from build123d import *
from build123d.topology import SkipClean

# Parameters (mm, degrees)
ESQUISSE1_W             = 22
ESQUISSE1_H             = 25
EXTRUSION1_DEPTH        = 5
EXTRUSION2_DEPTH        = 22
EXTRUSION3_DEPTH        = 9
EXTRUSION4_DEPTH        = 7.7
ESQUISSE6_R             = 1.25
EXTRUSION5_DEPTH        = 36
ENL_V_MAT_EXTRU_2_DEPTH = 6.678544503


with BuildPart() as part:
    # Esquisse1 → Extrusion1 (new, symmetric)
    with BuildSketch(Plane.XY):
        with Locations((11, 12.5)):
            Rectangle(ESQUISSE1_W, ESQUISSE1_H)
    extrude(amount=EXTRUSION1_DEPTH, both=True)

    # Esquisse2 → Extrusion2 (add)
    with BuildSketch(Plane.ZY):
        with BuildLine():
            Line((-5, 0), (5, 0))
            ThreePointArc((5, 0), (5.353553391, -0.146446609), (5.5, -0.5))
            Line((5.5, -0.5), (5.5, -10))
            Line((5.5, -10), (-5.5, -10))
            Line((-5.5, -10), (-5.5, -0.5))
            ThreePointArc((-5.5, -0.5), (-5.353553391, -0.146446609), (-5, 0))
        make_face()
    extrude(amount=-EXTRUSION2_DEPTH)

    # Esquisse4 → Extrusion3 (add)
    with BuildSketch(Plane(origin=(22, 0, 0), x_dir=(0, 0, -1), z_dir=(1, 0, 0))):
        with BuildLine():
            Line((5.5, -6), (5.5, -0.5))
            ThreePointArc((5.5, -0.5), (5.353553391, -0.146446609), (5, 0))
            Line((5, 0), (-5, 0))
            ThreePointArc((-5, 0), (-5.353553391, -0.146446609), (-5.5, -0.5))
            Line((-5.5, -0.5), (-5.5, -6))
            ThreePointArc((-5.5, -6), (-4.328427125, -8.828427125), (-1.5, -10))
            Line((-1.5, -10), (1.5, -10))
            ThreePointArc((1.5, -10), (4.328427125, -8.828427125), (5.5, -6))
        make_face()
    extrude(amount=EXTRUSION3_DEPTH)

    # Esquisse5 → Extrusion4 (add)
    with BuildSketch(Plane(origin=(22, 0, 0), x_dir=(0, 0, -1), z_dir=(1, 0, 0))):
        with BuildLine():
            Line((-2.42899156, 18.95), (-2.42899156, 14.05))
            ThreePointArc((-2.42899156, 14.05), (0, 13.05), (2.42899156, 14.05))
            Line((2.42899156, 14.05), (2.42899156, 18.95))
            ThreePointArc((2.42899156, 18.95), (0, 19.95), (-2.42899156, 18.95))
        make_face()
    extrude(amount=EXTRUSION4_DEPTH)

    # Esquisse6 → Extrusion5 (add)
    with BuildSketch(Plane.ZY):
        with Locations(Location((0, 16.5, 0), (0, 0, 180))):
            Circle(ESQUISSE6_R)
    extrude(amount=EXTRUSION5_DEPTH)

    # Esquisse7 → Révolution1 (revolve)
    with BuildSketch(Plane.XY, mode=Mode.PRIVATE) as r_volution1_sk:
        Polygon((-2, 17.75), (-2, 22.75), (-6, 22.75), (-6.821455497, 21.75), (-13.321455497, 21.75), (-13.321455497, 23.25), (-20, 23.25), (-20, 21.75), (-24.5, 21.75), (-24.5, 18.75), (-29, 18.75), (-29, 19.75), (-36, 19.75), (-36, 17.75), align=None)
    revolve(r_volution1_sk.sketch.rotate(Axis((0, 16.5, 0), (-1, 0, 0)), 90), axis=Axis((0, 16.5, 0), (-1, 0, 0)))

    # Esquisse8 → Enlèv. mat.-Extru.2 (cut)
    with SkipClean():  # the faces are left unmerged after this step: merging them gives an invalid solid
        with BuildSketch(Plane.ZY.offset(20)):
            with BuildLine():
                ThreePointArc((-3.202562433, 20.660059358), (-3.544451524, 21.369801094), (-3.707751714, 22.140485549))
                ThreePointArc((-3.707751714, 22.140485549), (-4.620864959, 21.420376716), (-5.396827126, 20.554227049))
                ThreePointArc((-5.396827126, 20.554227049), (-4.63790237, 20.342910474), (-3.951001573, 19.957178991))
                ThreePointArc((-3.951001573, 19.957178991), (-3.594006079, 20.326959668), (-3.202562433, 20.660059358))
            make_face()
            with BuildLine():
                ThreePointArc((-1.233637785, 21.603002823), (-1.25729104, 22.390442983), (-1.093007579, 23.160918438))
                ThreePointArc((-1.093007579, 23.160918438), (-2.220072686, 22.874462901), (-3.281244207, 22.398808054))
                ThreePointArc((-3.281244207, 22.398808054), (-2.673882137, 21.897078248), (-2.203258163, 21.26530728))
                ThreePointArc((-2.203258163, 21.26530728), (-1.7267232, 21.457915589), (-1.233637785, 21.603002823))
            make_face()
            with BuildLine():
                ThreePointArc((0.948594043, 21.663590741), (1.247266486, 22.392573768), (1.710727497, 23.029618016))
                ThreePointArc((1.710727497, 23.029618016), (0.564590324, 23.226346539), (-0.598304355, 23.223431557))
                ThreePointArc((-0.598304355, 23.223431557), (-0.247523392, 22.518042162), (-0.0745514, 21.749470648))
                ThreePointArc((-0.0745514, 21.749470648), (0.439125807, 21.731602864), (0.948594043, 21.663590741))
            make_face()
            with BuildLine():
                ThreePointArc((4.218662246, 21.769287319), (3.251630537, 22.415183754), (2.188087756, 22.885512663))
                ThreePointArc((2.188087756, 22.885512663), (2.221634397, 22.098431915), (2.067045976, 21.325952852))
                ThreePointArc((2.067045976, 21.325952852), (2.529045974, 21.100698476), (2.966805343, 20.83134691))
                ThreePointArc((2.966805343, 20.83134691), (3.536160307, 21.375825016), (4.218662246, 21.769287319))
            make_face()
            with BuildLine():
                ThreePointArc((5.997151968, 19.597848975), (5.376434291, 20.581231961), (4.596139615, 21.44348062))
                ThreePointArc((4.596139615, 21.44348062), (4.306651415, 20.710801929), (3.851232325, 20.067983966))
                ThreePointArc((3.851232325, 20.067983966), (4.181671115, 19.674291525), (4.472029047, 19.250173849))
                ThreePointArc((4.472029047, 19.250173849), (5.213619885, 19.516001823), (5.997151968, 19.597848975))
            make_face()
            with BuildLine():
                ThreePointArc((6.738679632, 16.8907644), (6.571603712, 18.041598084), (6.209477181, 19.146675867))
                ThreePointArc((6.209477181, 19.146675867), (5.647009279, 18.595086036), (4.969505618, 18.193078237))
                ThreePointArc((4.969505618, 18.193078237), (5.111247332, 17.699020732), (5.203998302, 17.193470745))
                ThreePointArc((5.203998302, 17.193470745), (5.98959722, 17.134684515), (6.738679632, 16.8907644))
            make_face()
            with BuildLine():
                ThreePointArc((6.315028369, 14.116113111), (6.63048315, 15.235407894), (6.74913973, 16.392236812))
                ThreePointArc((6.74913973, 16.392236812), (6.010947937, 16.117110733), (5.228506242, 16.0254239))
                ThreePointArc((5.228506242, 16.0254239), (5.15704245, 15.516428362), (5.036148973, 15.016860249))
                ThreePointArc((5.036148973, 15.016860249), (5.729918783, 14.643624489), (6.315028369, 14.116113111))
            make_face()
            with BuildLine():
                ThreePointArc((4.79945133, 11.753657521), (5.542891816, 12.647877167), (6.121814706, 13.656430992))
                ThreePointArc((6.121814706, 13.656430992), (5.335539089, 13.705340464), (4.583450638, 13.939828082))
                ThreePointArc((4.583450638, 13.939828082), (4.311138079, 13.503904463), (3.997503735, 13.09669809))
                ThreePointArc((3.997503735, 13.09669809), (4.479485333, 12.473548654), (4.79945133, 11.753657521))
            make_face()
            with BuildLine():
                ThreePointArc((2.454005555, 10.211887665), (3.496884131, 10.726413474), (4.435972305, 11.412304086))
                ThreePointArc((4.435972305, 11.412304086), (3.737567061, 11.776792217), (3.145874779, 12.296909248))
                ThreePointArc((3.145874779, 12.296909248), (2.719798768, 12.009432702), (2.267653785, 11.76499775))
                ThreePointArc((2.267653785, 11.76499775), (2.454508175, 10.999682835), (2.454005555, 10.211887665))
            make_face()
            with BuildLine():
                ThreePointArc((-4.617734942, 18.997803837), (-5.218744139, 19.507126354), (-5.681391894, 20.144761467))
                ThreePointArc((-5.681391894, 20.144761467), (-6.222667702, 19.115512697), (-6.579249607, 18.008633356))
                ThreePointArc((-6.579249607, 18.008633356), (-5.799987148, 18.124268567), (-5.015580917, 18.051273047))
                ThreePointArc((-5.015580917, 18.051273047), (-4.839852657, 18.534287653), (-4.617734942, 18.997803837))
            make_face()
            with BuildLine():
                ThreePointArc((-5.234459128, 16.90365534), (-5.990668481, 17.124492149), (-6.672667801, 17.518825015))
                ThreePointArc((-6.672667801, 17.518825015), (-6.748514668, 16.358402772), (-6.624060061, 15.202183251))
                ThreePointArc((-6.624060061, 15.202183251), (-5.959201458, 15.624775868), (-5.212920756, 15.8771379))
                ThreePointArc((-5.212920756, 15.8771379), (-5.248844742, 16.389868823), (-5.234459128, 16.90365534))
            make_face()
            with BuildLine():
                ThreePointArc((-4.946097778, 14.739711168), (-5.72675182, 14.633877579), (-6.510178827, 14.716724463))
                ThreePointArc((-6.510178827, 14.716724463), (-6.10748214, 13.625776294), (-5.523510351, 12.620137451))
                ThreePointArc((-5.523510351, 12.620137451), (-5.088015698, 13.276617374), (-4.508899238, 13.810701269))
                ThreePointArc((-4.508899238, 13.810701269), (-4.750263886, 14.264492673), (-4.946097778, 14.739711168))
            make_face()
            with BuildLine():
                ThreePointArc((-2.001435869, 11.646469897), (-2.445145697, 10.995514391), (-3.030927918, 10.46875005))
                ThreePointArc((-3.030927918, 10.46875005), (-1.950738753, 10.0380252), (-0.812650054, 9.799097084))
                ThreePointArc((-0.812650054, 9.799097084), (-1.00910691, 10.562003491), (-1.018504045, 11.349742772))
                ThreePointArc((-1.018504045, 11.349742772), (-1.517241252, 11.4740196), (-2.001435869, 11.646469897))
            make_face()
            with BuildLine():
                ThreePointArc((-0.315760074, 9.757389558), (0.846233411, 9.803255342), (1.983109992, 10.047886024))
                ThreePointArc((1.983109992, 10.047886024), (1.493335733, 10.664929505), (1.164348592, 11.380742988))
                ThreePointArc((1.164348592, 11.380742988), (0.658181542, 11.291420822), (0.145705895, 11.252022314))
                ThreePointArc((0.145705895, 11.252022314), (0.005124254, 10.476871823), (-0.315760074, 9.757389558))
            make_face()
            with BuildLine():
                ThreePointArc((-3.802511188, 12.880136927), (-4.472627743, 12.465932528), (-5.22202079, 12.222968452))
                ThreePointArc((-5.22202079, 12.222968452), (-4.410410464, 11.390129206), (-3.467895523, 10.708955134))
                ThreePointArc((-3.467895523, 10.708955134), (-3.3370658, 11.485811019), (-3.02524808, 12.20926882))
                ThreePointArc((-3.02524808, 12.20926882), (-3.43031925, 12.525656049), (-3.802511188, 12.880136927))
            make_face()
        extrude(amount=-ENL_V_MAT_EXTRU_2_DEPTH, mode=Mode.SUBTRACT)


solid = part.part
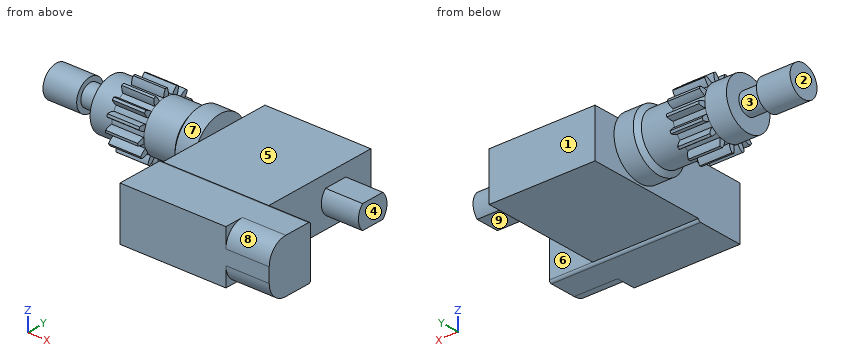
The listing builds one solid part. Answer for the finished solid, in the listing's coordinates (mm). Face numbers are marked on the shaded views. A direction names the side the tool comes from. Give positions to 0.01 mm unless a question says otherwise; leave off trailing zeros. Order: outer loops, then holes, each group sorted by start corner. A loop starts at its lowest first (then second) coordinate and runs counter-clockwise, first axis right, second up. Notation, with made-up numbers: (-35, -35.75) - (-30, -35.75) arc R26 cw to (-30, -19.75) - close; hole circle Ø10 at (76, -18). An arc over 180 degrees is marked (long way). One line per item, written item: value. Start each with the question number.
1) The mould has two halves that part along X. Classify the marked faces 1, 2, 3 and 4: released by +X, released by -X, zero draft, split by the parting line, or undercut.
2) Given pin 1 Ø1.4 at (y, z) = (15, -5.5) entering from +X; pin 2 Ø0.5 at (y, z) = (21.5, -3.5) entering from -X; pin 3 Ø17.5 at (x, y) = (12.5, 16.5) entering from -Z, each flat-ended and moving along its own axis, determine where each tip first touches the part or whether it passes through.
3) Find the intervals of material crossed by L1, parallel to X at y = 12, z = -3; L2, parallel to X at y = 21, z = 0.75; L3, parallel to X at y = -6, z = -2.5, in increasing order.
4) A cutting plane is placed at A-A on x = 11.5. Give the vertices of the cut face in (y, z).
5) A tool of negligible diameter and unlimited length cuts with its end or side. For the marked faces 5, 6, 7, 8 and 9, from which of +Z, -Z, +X, -X, +Y, -Y can it reach the whole face along a straight path? Write none if from no direction.
6) A cutting plane is placed at B-B on x = -5. Give the vertices of the cut face in (y, z), then the cut area to 3 significant figures.
Answer sheet:
1. face 1: zero draft
1. face 2: released by -X
1. face 3: undercut
1. face 4: released by +X
2. pin 1: stops at x = 22
2. pin 2: stops at x = -20
2. pin 3: stops at z = -5
3. L1: x = -20 to -13.32, -6.69 to -2, 0 to 22
3. L2: x = -24.5 to -2, 0 to 22
3. L3: x = 0 to 31
4. outline: (-10, -5.5) - (-0.5, -5.5) arc R0.5 ccw to (0, -5) - (25, -5) - (25, 5) - (0, 5) arc R0.5 ccw to (-0.5, 5.5) - (-10, 5.5) - close
5. face 5: +Z, +X, +Y
5. face 6: +Z, -Z, +X
5. face 7: none
5. face 8: +Z, +X, -Y
5. face 9: -Z, +X, +Y
6. outline: circle Ø12.5 at (16.5, 0)
6. area: 123 mm2
